Geometry check sheet. Reference: the model listing, model coordinates, mm. Round coordinates to 2 decimals unless told otherwise and drop trailing zeros. Order: outer loops, then holes, each group sorted by start corner. A loop starts at its lowest first (then second) coordinate and runs counter-clockwise, first axis right, second up.
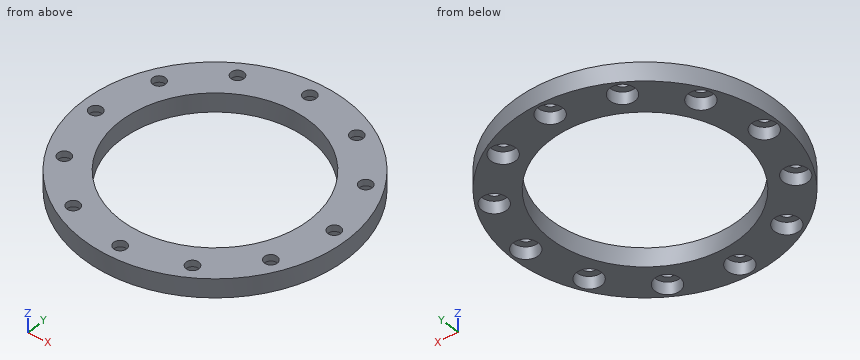
```python
from build123d import *

# Parameters (mm, degrees)
SKETCH1_R           = 35
SKETCH1_R_2         = 25
BOSS_EXTRUDE1_DEPTH = 5
CUT_EXTRUDE1_REACH  = 51.749
SKETCH2_R           = 1.7
SKETCH3_R           = 3.3
CUT_EXTRUDE2_DEPTH  = 3.3
CIRPATTERN1_COUNT   = 12


with BuildPart() as part:
    # Sketch1 → Boss-Extrude1 (new body)
    with BuildSketch(Plane.XY):
        Circle(SKETCH1_R)
        Circle(SKETCH1_R_2, mode=Mode.SUBTRACT)
    extrude(amount=BOSS_EXTRUDE1_DEPTH)

    # Sketch2 → Cut-Extrude1 (cut, up to next)
    with BuildSketch(Plane.XY.offset(5), mode=Mode.PRIVATE) as cut_extrude1_sk1:
        with Locations((0, 31)):
            Circle(SKETCH2_R)
    cut_extrude1_tool1 = extrude(cut_extrude1_sk1.sketch, amount=-CUT_EXTRUDE1_REACH, mode=Mode.PRIVATE) & part.part
    # Sketch2 → Cut-Extrude1 (cut, up to next)
    with BuildSketch(Plane.XY.offset(5), mode=Mode.PRIVATE) as cut_extrude1_sk2:
        with Locations((15.5, 26.846787517)):
            Circle(SKETCH2_R)
    cut_extrude1_tool2 = extrude(cut_extrude1_sk2.sketch, amount=-CUT_EXTRUDE1_REACH, mode=Mode.PRIVATE) & part.part
    # Sketch2 → Cut-Extrude1 (cut, up to next)
    with BuildSketch(Plane.XY.offset(5), mode=Mode.PRIVATE) as cut_extrude1_sk3:
        with Locations((26.846787517, 15.5)):
            Circle(SKETCH2_R)
    cut_extrude1_tool3 = extrude(cut_extrude1_sk3.sketch, amount=-CUT_EXTRUDE1_REACH, mode=Mode.PRIVATE) & part.part
    # Sketch2 → Cut-Extrude1 (cut, up to next)
    with BuildSketch(Plane.XY.offset(5), mode=Mode.PRIVATE) as cut_extrude1_sk4:
        with Locations((31, 0)):
            Circle(SKETCH2_R)
    cut_extrude1_tool4 = extrude(cut_extrude1_sk4.sketch, amount=-CUT_EXTRUDE1_REACH, mode=Mode.PRIVATE) & part.part
    # Sketch2 → Cut-Extrude1 (cut, up to next)
    with BuildSketch(Plane.XY.offset(5), mode=Mode.PRIVATE) as cut_extrude1_sk5:
        with Locations((26.846787517, -15.5)):
            Circle(SKETCH2_R)
    cut_extrude1_tool5 = extrude(cut_extrude1_sk5.sketch, amount=-CUT_EXTRUDE1_REACH, mode=Mode.PRIVATE) & part.part
    # Sketch2 → Cut-Extrude1 (cut, up to next)
    with BuildSketch(Plane.XY.offset(5), mode=Mode.PRIVATE) as cut_extrude1_sk6:
        with Locations((15.5, -26.846787517)):
            Circle(SKETCH2_R)
    cut_extrude1_tool6 = extrude(cut_extrude1_sk6.sketch, amount=-CUT_EXTRUDE1_REACH, mode=Mode.PRIVATE) & part.part
    # Sketch2 → Cut-Extrude1 (cut, up to next)
    with BuildSketch(Plane.XY.offset(5), mode=Mode.PRIVATE) as cut_extrude1_sk7:
        with Locations((0, -31)):
            Circle(SKETCH2_R)
    cut_extrude1_tool7 = extrude(cut_extrude1_sk7.sketch, amount=-CUT_EXTRUDE1_REACH, mode=Mode.PRIVATE) & part.part
    # Sketch2 → Cut-Extrude1 (cut, up to next)
    with BuildSketch(Plane.XY.offset(5), mode=Mode.PRIVATE) as cut_extrude1_sk8:
        with Locations((-15.5, -26.846787517)):
            Circle(SKETCH2_R)
    cut_extrude1_tool8 = extrude(cut_extrude1_sk8.sketch, amount=-CUT_EXTRUDE1_REACH, mode=Mode.PRIVATE) & part.part
    # Sketch2 → Cut-Extrude1 (cut, up to next)
    with BuildSketch(Plane.XY.offset(5), mode=Mode.PRIVATE) as cut_extrude1_sk9:
        with Locations((-26.846787517, -15.5)):
            Circle(SKETCH2_R)
    cut_extrude1_tool9 = extrude(cut_extrude1_sk9.sketch, amount=-CUT_EXTRUDE1_REACH, mode=Mode.PRIVATE) & part.part
    # Sketch2 → Cut-Extrude1 (cut, up to next)
    with BuildSketch(Plane.XY.offset(5), mode=Mode.PRIVATE) as cut_extrude1_sk10:
        with Locations((-31, 0)):
            Circle(SKETCH2_R)
    cut_extrude1_tool10 = extrude(cut_extrude1_sk10.sketch, amount=-CUT_EXTRUDE1_REACH, mode=Mode.PRIVATE) & part.part
    # Sketch2 → Cut-Extrude1 (cut, up to next)
    with BuildSketch(Plane.XY.offset(5), mode=Mode.PRIVATE) as cut_extrude1_sk11:
        with Locations((-26.846787517, 15.5)):
            Circle(SKETCH2_R)
    cut_extrude1_tool11 = extrude(cut_extrude1_sk11.sketch, amount=-CUT_EXTRUDE1_REACH, mode=Mode.PRIVATE) & part.part
    # Sketch2 → Cut-Extrude1 (cut, up to next)
    with BuildSketch(Plane.XY.offset(5), mode=Mode.PRIVATE) as cut_extrude1_sk12:
        with Locations((-15.5, 26.846787517)):
            Circle(SKETCH2_R)
    cut_extrude1_tool12 = extrude(cut_extrude1_sk12.sketch, amount=-CUT_EXTRUDE1_REACH, mode=Mode.PRIVATE) & part.part
    add(cut_extrude1_tool1.solids().sort_by_distance((0, 31, 5))[0], mode=Mode.SUBTRACT)
    add(cut_extrude1_tool2.solids().sort_by_distance((15.5, 26.846788, 5))[0], mode=Mode.SUBTRACT)
    add(cut_extrude1_tool3.solids().sort_by_distance((26.846788, 15.5, 5))[0], mode=Mode.SUBTRACT)
    add(cut_extrude1_tool4.solids().sort_by_distance((31, 0, 5))[0], mode=Mode.SUBTRACT)
    add(cut_extrude1_tool5.solids().sort_by_distance((26.846788, -15.5, 5))[0], mode=Mode.SUBTRACT)
    add(cut_extrude1_tool6.solids().sort_by_distance((15.5, -26.846788, 5))[0], mode=Mode.SUBTRACT)
    add(cut_extrude1_tool7.solids().sort_by_distance((0, -31, 5))[0], mode=Mode.SUBTRACT)
    add(cut_extrude1_tool8.solids().sort_by_distance((-15.5, -26.846788, 5))[0], mode=Mode.SUBTRACT)
    add(cut_extrude1_tool9.solids().sort_by_distance((-26.846788, -15.5, 5))[0], mode=Mode.SUBTRACT)
    add(cut_extrude1_tool10.solids().sort_by_distance((-31, 0, 5))[0], mode=Mode.SUBTRACT)
    add(cut_extrude1_tool11.solids().sort_by_distance((-26.846788, 15.5, 5))[0], mode=Mode.SUBTRACT)
    add(cut_extrude1_tool12.solids().sort_by_distance((-15.5, 26.846788, 5))[0], mode=Mode.SUBTRACT)

    # Sketch3 → Cut-Extrude2 (cut)
    with BuildSketch(Plane(origin=(0, 0, 0), x_dir=(-1, 0, 0), z_dir=(0, 0, -1))):
        with Locations((0, 31)):
            Circle(SKETCH3_R)
    cut_extrude2 = extrude(amount=-CUT_EXTRUDE2_DEPTH, mode=Mode.SUBTRACT)

    # CirPattern1: Cut-Extrude2 ×12 about axis
    cirpattern1_axis = Axis((0, 0, 0), (0, 0, 1))
    for i in range(1, CIRPATTERN1_COUNT):
        add(cut_extrude2.rotate(cirpattern1_axis, i * 360 / CIRPATTERN1_COUNT), mode=Mode.SUBTRACT)


solid = part.part
```
(1) Sectioned sample at A-A, the plane x = 0. Record the cut outline in (y, z), and give its area (3 significant figures).
Returned:
outline: (-35, 0) - (-34.3, 0) - (-34.3, 3.3) - (-32.7, 3.3) - (-32.7, 5) - (-35, 5) - close; (-29.3, 3.3) - (-27.7, 3.3) - (-27.7, 0) - (-25, 0) - (-25, 5) - (-29.3, 5) - close; (25, 0) - (27.7, 0) - (27.7, 3.3) - (29.3, 3.3) - (29.3, 5) - (25, 5) - close; (32.7, 3.3) - (34.3, 3.3) - (34.3, 0) - (35, 0) - (35, 5) - (32.7, 5) - close
area: 44.9 mm2
(2) Depth check by flat-ended pin: P1, Ø3.5, axis at x = 27.5, y = -16, coming from the -Z side; P2, Ø1, axis at x = 26, z = 0.5, coming from the +Y side; P3, Ø8, axis at x = 9.5, y = 17, coming from the -Z side; P4, Ø1.5, axis at x = 11, z = 1.5, coming from the +Y side. Enter the tip coordinate at first touch or a pass-through.
Returned:
P1: stops at z = 3.3
P2: stops at y = 23.97
P3: passes through
P4: stops at y = 33.47
(3) Sectioned sample at B-B, the plane y = 31. Record the cut outline in (x, z).
Returned:
outline: (-16.25, 0) - (-3.3, 0) - (-3.3, 3.3) - (-1.7, 3.3) - (-1.7, 5) - (-16.25, 5) - close; (1.7, 3.3) - (3.3, 3.3) - (3.3, 0) - (16.25, 0) - (16.25, 5) - (1.7, 5) - close
(4) Material ranges on line 1 (Y direction, x = -16, z = 1.4); line 2 (X direction, y = -1.5, z = 2.35); line 3 (X direction, y = 15, z = 0.75), recorded low to high.
Returned:
line 1: y = -31.13 to -30.11, -23.58 to -19.21, 19.21 to 23.58, 30.11 to 31.13
line 2: x = -34.97 to -33.94, -28.06 to -24.95, 24.95 to 28.06, 33.94 to 34.97
line 3: x = -31.62 to -30.11, -23.58 to -20, 20 to 23.58, 30.11 to 31.62
